```python
from build123d import *

# Parameters (mm, degrees)
SKETCH1_W           = 65.122
SKETCH1_H           = 27.725
BOSS_EXTRUDE1_DEPTH = 50
SKETCH3_W           = 65.122
SKETCH3_H           = 30
CUT_EXTRUDE1_DEPTH  = 25.272
CUT_EXTRUDE2_DEPTH  = 87.657662725
CUT_EXTRUDE3_DEPTH  = 87.657662725
SKETCH6_W           = 5
SKETCH6_H           = 10
BOSS_EXTRUDE2_DEPTH = 15
CUT_EXTRUDE5_DEPTH  = 15
SKETCH9_R           = 1.5
CUT_EXTRUDE6_DEPTH  = 83.877473568
SKETCH10_R          = 1.575
CUT_EXTRUDE7_DEPTH  = 86.904300637


with BuildPart() as part:
    # Sketch1 → Boss-Extrude1 (new body)
    with BuildSketch(Plane.XY):
        with Locations((32.561, 13.8625)):
            Rectangle(SKETCH1_W, SKETCH1_H)
    extrude(amount=BOSS_EXTRUDE1_DEPTH)

    # Sketch3 → Cut-Extrude1 (cut)
    with BuildSketch(Plane(origin=(0, 27.725, 0), x_dir=(1, 0, 0), z_dir=(0, 1, 0))):
        with Locations((32.561, -25)):
            Rectangle(SKETCH3_W, SKETCH3_H)
    extrude(amount=-CUT_EXTRUDE1_DEPTH, mode=Mode.SUBTRACT)

    # Sketch4 → Cut-Extrude2 (cut, through all)
    with BuildSketch(Plane.XY.offset(50)):
        Polygon((0, 27.725), (0, 5), (46.655, 27.725), align=None)
    extrude(amount=-CUT_EXTRUDE2_DEPTH, mode=Mode.SUBTRACT)

    # Sketch5 → Cut-Extrude3 (cut, through all)
    with BuildSketch(Plane.XY.offset(50)):
        Polygon((46.655, 27.725), (65.122, 0), (65.122, 27.725), align=None)
    extrude(amount=-CUT_EXTRUDE3_DEPTH, mode=Mode.SUBTRACT)

    # Sketch6 → Boss-Extrude2 (add)
    with BuildSketch(Plane(origin=(0, 2.453, 0), x_dir=(1, 0, 0), z_dir=(0, 1, 0))):
        with Locations((57.5, -25)):
            Rectangle(SKETCH6_W, SKETCH6_H)
    extrude(amount=BOSS_EXTRUDE2_DEPTH)

    # Sketch7 → Cut-Extrude5 (cut)
    with BuildSketch(Plane(origin=(60, 0, 0), x_dir=(0, 0, -1), z_dir=(1, 0, 0))):
        with BuildLine():
            Line((-30, 15.453), (-30, 17.453))
            Line((-30, 17.453), (-24.889040711, 17.831001858))
            Line((-24.889040711, 17.831001858), (-20, 17.453))
            Line((-20, 17.453), (-20, 15.453))
            ThreePointArc((-20, 15.453), (-25, 17.453), (-30, 15.453))
        make_face()
    extrude(amount=-CUT_EXTRUDE5_DEPTH, mode=Mode.SUBTRACT)

    # Sketch9 → Cut-Extrude6 (cut, through all)
    with BuildSketch(Plane(origin=(60, 0, 0), x_dir=(0, 0, -1), z_dir=(1, 0, 0))):
        with Locations((-25, 12.453)):
            Circle(SKETCH9_R)
    extrude(amount=-CUT_EXTRUDE6_DEPTH, mode=Mode.SUBTRACT)

    # Sketch10 → Cut-Extrude7 (cut, through all)
    with BuildSketch(Plane(origin=(0, 2.453, 0), x_dir=(1, 0, 0), z_dir=(0, 1, 0))):
        with Locations(Location((46.10608811, -35, 0), (0, 0, 270))):
            Circle(SKETCH10_R)
        with Locations(Location((46.10608811, -13, 0), (0, 0, 270))):
            Circle(SKETCH10_R)
    extrude(amount=-CUT_EXTRUDE7_DEPTH, mode=Mode.SUBTRACT)


solid = part.part
```
Model file for the job. Use its own axes, mm. A direction names the side the tool comes from. Coordinates: 2 decimals unless noted, no trailing zeros. Write each loop counter-clockwise with the first axis right and the second up, starting at its lowest first coordinate (ties: lowest second). Pieces come first, ordered by that corner, then holes. Notation, with made-up numbers: (7, -8) - (29, -8) arc R10 cw to (29, 4) - close; hole circle Ø7 at (-14.5, -15). An arc over 180 degrees is marked (long way). One line per item, written item: value. Start each with the question number.
1. Slice it at A-A (z = 25). Write the cut outline in (x, y), plus the area to 3 significant figures.
2. Tool access for faces 1 (the flat face through (55, 10, 25)), 2 (the flat face through (38, 10, 40)), 3 (the flat face through (63.97, 1.73, 25.35)), 4 (the flat face through (32, 11, 0)): list every direction of +Z, -Z, +X, -X, +Y, -Y with a clear straight run to the whole face (end or side of a thin tool).
3. Probe line 1 (Z direction, x = 30, y = 4.75); line 2 (Y direction, x = 57.5, z = 16); line 3 (X direction, y = 1, z = 13). List the from-to ranges inside material, lowest first. Write a range as from..to.
4. Mould opens along Z. For faces 5 (the flat face through (23.001, 16.203, 45.07)), 6 (the flat face through (57, 9, 20)), 7 (the flat face through (60, 10, 25)), 8 (the flat face through (32, 11, 50)) say: released by +Z, released by -Z, zero draft, split by the parting line, or undercut.
5. Slice it at D-D (z = 35). Write the cut outline in (x, y), plus the area to 3 significant figures.
6. Flat gauge pins, fed straight in: pin 1 (2.5 mm diameter, centred on x = 46.11, z = 35, fed in from +Y) (1 decimal); pin 2 (10 mm diameter, centred on x = 27.5, z = 11, fed in from +Y); pin 3 (8 mm diameter, centred on x = 19.5, z = 26.5, fed in from +Y); pin 4 (5 mm diameter, centred on y = 6.5, z = 24.5, fed in from -X). Where does each tip first touch, or does it go through?
7. Slice it at C-C (y = 8). Write the cut outline in (x, z).
8. Slice it at B-B (x = 58). Write the cut outline in (y, z), plus the area to 3 significant figures.
Answers below:
1. outline: (0, 0) - (65.12, 0) - (63.49, 2.45) - (60, 2.45) - (60, 10.95) - (55, 10.95) - (55, 2.45) - (0, 2.45) - close; (55, 13.95) - (60, 13.95) - (60, 17.45) - (55, 17.45) - close
1. area: 218 mm^2
2. face 1: -X, +Y
2. face 2: +X, -X, +Y
2. face 3: +X, +Y
2. face 4: -Z, +X, -X, +Y, -Y
3. line 1: z = 0..10, 40..50
3. line 2: y = 0..2.45
3. line 3: x = 0..44.53, 47.68..64.46
4. face 5: zero draft
4. face 6: undercut
4. face 7: undercut
4. face 8: released by +Z
5. outline: (0, 0) - (44.53, 0) - (44.53, 2.45) - (0, 2.45) - close; (47.68, 0) - (65.12, 0) - (63.49, 2.45) - (47.68, 2.45) - close
5. area: 150 mm^2
6. pin 1: passes through
6. pin 2: stops at y = 20.78
6. pin 3: stops at y = 2.45
6. pin 4: stops at x = 55
7. outline: (6.16, 0) - (59.79, 0) - (59.79, 10) - (6.16, 10) - close; (6.16, 40) - (59.79, 40) - (59.79, 50) - (6.16, 50) - close; (55, 20) - (60, 20) - (60, 30) - (55, 30) - close
8. outline: (0, 0) - (10.69, 0) - (10.69, 10) - (2.45, 10) - (2.45, 20) - (15.45, 20) arc R7.25 ccw to (15.45, 30) - (2.45, 30) - (2.45, 40) - (10.69, 40) - (10.69, 50) - (0, 50) - close; hole circle Ø3 at (12.45, 25)
8. area: 424 mm^2
